```python
from build123d import *

# Parameters (mm, degrees)
F1_DEPTH = 6.35


with BuildPart() as f1:
    # F0 (on Front) → F1 (new body)
    with BuildSketch(Plane.XZ):
        with BuildLine():
            Line((68.58, 18.1031430027), (30.48, 25.4))
            Line((30.48, 25.4), (-30.48, 25.4))
            Line((-30.48, 25.4), (-68.58, 18.1031430027))
            Line((-68.58, 18.1031430027), (-68.58, 17.78))
            ThreePointArc((-68.58, 17.78), (-65.5387583202, 17.5179693185), (-62.5871565312, 16.7396005675))
            Line((-62.5871565312, 16.7396005675), (-61.5696, 17.3270871047))
            Line((-61.5696, 17.3270871047), (-59.9821, 16.4105435523))
            Line((-59.9821, 16.4105435523), (-59.9821, 15.5629211779))
            ThreePointArc((-59.9821, 15.5629211779), (-53.2666224823, 9.0348696172), (-50.8, 0))
            ThreePointArc((-50.8, 0), (-53.2666224823, -9.0348696172), (-59.9821, -15.5629211779))
            Line((-59.9821, -15.5629211779), (-59.9821, -16.4105435523))
            Line((-59.9821, -16.4105435523), (-61.5696, -17.3270871047))
            Line((-61.5696, -17.3270871047), (-62.5871565312, -16.7396005675))
            ThreePointArc((-62.5871565312, -16.7396005675), (-65.5387583202, -17.5179693185), (-68.58, -17.78))
            Line((-68.58, -17.78), (-68.58, -18.1031430027))
            Line((-68.58, -18.1031430027), (-30.48, -25.4))
            Line((-30.48, -25.4), (30.48, -25.4))
            Line((30.48, -25.4), (68.58, -18.1031430027))
            Line((68.58, -18.1031430027), (68.58, -17.78))
            ThreePointArc((68.58, -17.78), (50.8, 0), (68.58, 17.78))
            Line((68.58, 17.78), (68.58, 18.1031430027))
        make_face()
        Polygon((-30.48, -18.4869128953), (-28.8925, -19.4034564477), (-28.8925, -21.2365435523), (-30.48, -22.1530871047), (-32.0675, -21.2365435523), (-32.0675, -19.4034564477), align=None, mode=Mode.SUBTRACT)
        Polygon((-19.05, -15.9469128953), (-17.4625, -16.8634564477), (-17.4625, -18.6965435523), (-19.05, -19.6130871047), (-20.6375, -18.6965435523), (-20.6375, -16.8634564477), align=None, mode=Mode.SUBTRACT)
        Polygon((-48.1514023938, -5.9139128953), (-46.5639023938, -6.8304564477), (-46.5639023938, -8.6635435523), (-48.1514023938, -9.5800871047), (-49.7389023938, -8.6635435523), (-49.7389023938, -6.8304564477), align=None, mode=Mode.SUBTRACT)
        Polygon((0, -18.4869128953), (1.5875, -19.4034564477), (1.5875, -21.2365435523), (0, -22.1530871047), (-1.5875, -21.2365435523), (-1.5875, -19.4034564477), align=None, mode=Mode.SUBTRACT)
        Polygon((30.48, -22.1530871047), (28.8925, -21.2365435523), (28.8925, -19.4034564477), (30.48, -18.4869128953), (32.0675, -19.4034564477), (32.0675, -21.2365435523), align=None, mode=Mode.SUBTRACT)
        Polygon((19.05, -19.6130871047), (17.4625, -18.6965435523), (17.4625, -16.8634564477), (19.05, -15.9469128953), (20.6375, -16.8634564477), (20.6375, -18.6965435523), align=None, mode=Mode.SUBTRACT)
        Polygon((-48.1514023938, 9.5800871047), (-46.5639023938, 8.6635435523), (-46.5639023938, 6.8304564477), (-48.1514023938, 5.9139128953), (-49.7389023938, 6.8304564477), (-49.7389023938, 8.6635435523), align=None, mode=Mode.SUBTRACT)
        Polygon((-19.05, 19.6130871047), (-17.4625, 18.6965435523), (-17.4625, 16.8634564477), (-19.05, 15.9469128953), (-20.6375, 16.8634564477), (-20.6375, 18.6965435523), align=None, mode=Mode.SUBTRACT)
        Polygon((-30.48, 22.1530871047), (-28.8925, 21.2365435523), (-28.8925, 19.4034564477), (-30.48, 18.4869128953), (-32.0675, 19.4034564477), (-32.0675, 21.2365435523), align=None, mode=Mode.SUBTRACT)
        Polygon((19.05, 19.6130871047), (20.6375, 18.6965435523), (20.6375, 16.8634564477), (19.05, 15.9469128953), (17.4625, 16.8634564477), (17.4625, 18.6965435523), align=None, mode=Mode.SUBTRACT)
        Polygon((0, 22.1530871047), (1.5875, 21.2365435523), (1.5875, 19.4034564477), (0, 18.4869128953), (-1.5875, 19.4034564477), (-1.5875, 21.2365435523), align=None, mode=Mode.SUBTRACT)
        Polygon((30.48, 18.4869128953), (28.8925, 19.4034564477), (28.8925, 21.2365435523), (30.48, 22.1530871047), (32.0675, 21.2365435523), (32.0675, 19.4034564477), align=None, mode=Mode.SUBTRACT)
        with BuildLine():
            ThreePointArc((-62.5871565312, 16.7396005675), (-65.5387583202, 17.5179693185), (-68.58, 17.78))
            Line((-68.58, 17.78), (-68.58, 7.3323484187))
            Line((-68.58, 7.3323484187), (-62.23, 3.6661742094))
            Line((-62.23, 3.6661742094), (-62.23, -3.6661742094))
            Line((-62.23, -3.6661742094), (-68.58, -7.3323484187))
            Line((-68.58, -7.3323484187), (-68.58, -17.78))
            ThreePointArc((-68.58, -17.78), (-65.5387583202, -17.5179693185), (-62.5871565312, -16.7396005675))
            Line((-62.5871565312, -16.7396005675), (-63.1571, -16.4105435523))
            Line((-63.1571, -16.4105435523), (-63.1571, -14.5774564477))
            Line((-63.1571, -14.5774564477), (-61.5696, -13.6609128953))
            Line((-61.5696, -13.6609128953), (-59.9821, -14.5774564477))
            Line((-59.9821, -14.5774564477), (-59.9821, -15.5629211779))
            ThreePointArc((-59.9821, -15.5629211779), (-53.2666224823, -9.0348696172), (-50.8, 0))
            ThreePointArc((-50.8, 0), (-53.2666224823, 9.0348696172), (-59.9821, 15.5629211779))
            Line((-59.9821, 15.5629211779), (-59.9821, 14.5774564477))
            Line((-59.9821, 14.5774564477), (-61.5696, 13.6609128953))
            Line((-61.5696, 13.6609128953), (-63.1571, 14.5774564477))
            Line((-63.1571, 14.5774564477), (-63.1571, 16.4105435523))
            Line((-63.1571, 16.4105435523), (-62.5871565312, 16.7396005675))
        make_face()
        with BuildLine():
            Line((-68.58, 7.3323484187), (-68.58, 17.78))
            ThreePointArc((-68.58, 17.78), (-70.259720977, 17.7004784523), (-71.9244167559, 17.4626251338))
            ThreePointArc((-71.9244167559, 17.4626251338), (-86.36, 0), (-71.9244167559, -17.4626251338))
            ThreePointArc((-71.9244167559, -17.4626251338), (-70.259720977, -17.7004784523), (-68.58, -17.78))
            Line((-68.58, -17.78), (-68.58, -7.3323484187))
            Line((-68.58, -7.3323484187), (-74.93, -3.6661742094))
            Line((-74.93, -3.6661742094), (-74.93, 3.6661742094))
            Line((-74.93, 3.6661742094), (-68.58, 7.3323484187))
        make_face()
        Polygon((-74.9877976062, -9.5800871047), (-76.5752976062, -8.6635435523), (-76.5752976062, -6.8304564477), (-74.9877976062, -5.9139128953), (-73.4002976062, -6.8304564477), (-73.4002976062, -8.6635435523), align=None, mode=Mode.SUBTRACT)
        Polygon((-74.9877976062, 9.5800871047), (-73.4002976062, 8.6635435523), (-73.4002976062, 6.8304564477), (-74.9877976062, 5.9139128953), (-76.5752976062, 6.8304564477), (-76.5752976062, 8.6635435523), align=None, mode=Mode.SUBTRACT)
        with BuildLine():
            Line((68.58, -17.78), (68.58, 17.78))
            ThreePointArc((68.58, 17.78), (50.8, 0), (68.58, -17.78))
        make_face()
        Polygon((59.055, -1.8330871047), (57.4675, -0.9165435523), (57.4675, 0.9165435523), (59.055, 1.8330871047), (60.6425, 0.9165435523), (60.6425, -0.9165435523), align=None, mode=Mode.SUBTRACT)
        with BuildLine():
            ThreePointArc((71.9244167559, 17.4626251338), (70.259720977, 17.7004784523), (68.58, 17.78))
            Line((68.58, 17.78), (68.58, -17.78))
            ThreePointArc((68.58, -17.78), (70.259720977, -17.7004784523), (71.9244167559, -17.4626251338))
            ThreePointArc((71.9244167559, -17.4626251338), (82.2838704372, -11.3283862505), (86.36, 0))
            ThreePointArc((86.36, 0), (82.2838704372, 11.3283862505), (71.9244167559, 17.4626251338))
        make_face()
        Polygon((78.105, 1.8330871047), (79.6925, 0.9165435523), (79.6925, -0.9165435523), (78.105, -1.8330871047), (76.5175, -0.9165435523), (76.5175, 0.9165435523), align=None, mode=Mode.SUBTRACT)
        with BuildLine():
            ThreePointArc((-68.58, -17.78), (-70.259720977, -17.7004784523), (-71.9244167559, -17.4626251338))
            Line((-71.9244167559, -17.4626251338), (-68.58, -18.1031430027))
            Line((-68.58, -18.1031430027), (-68.58, -17.78))
        make_face()
        with BuildLine():
            Line((-68.58, 17.78), (-68.58, 18.1031430027))
            Line((-68.58, 18.1031430027), (-71.9244167559, 17.4626251338))
            ThreePointArc((-71.9244167559, 17.4626251338), (-70.259720977, 17.7004784523), (-68.58, 17.78))
        make_face()
        with BuildLine():
            Line((71.9244167559, 17.4626251338), (68.58, 18.1031430027))
            Line((68.58, 18.1031430027), (68.58, 17.78))
            ThreePointArc((68.58, 17.78), (70.259720977, 17.7004784523), (71.9244167559, 17.4626251338))
        make_face()
        with BuildLine():
            ThreePointArc((71.9244167559, -17.4626251338), (70.259720977, -17.7004784523), (68.58, -17.78))
            Line((68.58, -17.78), (68.58, -18.1031430027))
            Line((68.58, -18.1031430027), (71.9244167559, -17.4626251338))
        make_face()
        Polygon((-73.4002976062, 6.8304564477), (-73.4002976062, 8.6635435523), (-74.9877976062, 9.5800871047), (-76.5752976062, 8.6635435523), (-76.5752976062, 6.8304564477), (-74.9877976062, 5.9139128953), align=None)
        Polygon((-76.5752976062, -6.8304564477), (-76.5752976062, -8.6635435523), (-74.9877976062, -9.5800871047), (-73.4002976062, -8.6635435523), (-73.4002976062, -6.8304564477), (-74.9877976062, -5.9139128953), align=None)
        Polygon((-68.58, -7.3323484187), (-68.58, 7.3323484187), (-74.93, 3.6661742094), (-74.93, -3.6661742094), align=None)
        Polygon((-62.23, 3.6661742094), (-68.58, 7.3323484187), (-68.58, -7.3323484187), (-62.23, -3.6661742094), align=None)
        with BuildLine():
            ThreePointArc((-59.9821, 15.5629211779), (-61.260943207, 16.2036973454), (-62.5871565312, 16.7396005675))
            Line((-62.5871565312, 16.7396005675), (-63.1571, 16.4105435523))
            Line((-63.1571, 16.4105435523), (-63.1571, 14.5774564477))
            Line((-63.1571, 14.5774564477), (-61.5696, 13.6609128953))
            Line((-61.5696, 13.6609128953), (-59.9821, 14.5774564477))
            Line((-59.9821, 14.5774564477), (-59.9821, 15.5629211779))
        make_face()
        with BuildLine():
            Line((-61.5696, 17.3270871047), (-62.5871565312, 16.7396005675))
            ThreePointArc((-62.5871565312, 16.7396005675), (-61.260943207, 16.2036973454), (-59.9821, 15.5629211779))
            Line((-59.9821, 15.5629211779), (-59.9821, 16.4105435523))
            Line((-59.9821, 16.4105435523), (-61.5696, 17.3270871047))
        make_face()
        Polygon((-46.5639023938, 6.8304564477), (-46.5639023938, 8.6635435523), (-48.1514023938, 9.5800871047), (-49.7389023938, 8.6635435523), (-49.7389023938, 6.8304564477), (-48.1514023938, 5.9139128953), align=None)
        Polygon((-46.5639023938, -8.6635435523), (-46.5639023938, -6.8304564477), (-48.1514023938, -5.9139128953), (-49.7389023938, -6.8304564477), (-49.7389023938, -8.6635435523), (-48.1514023938, -9.5800871047), align=None)
        with BuildLine():
            Line((-63.1571, -16.4105435523), (-62.5871565312, -16.7396005675))
            ThreePointArc((-62.5871565312, -16.7396005675), (-61.260943207, -16.2036973454), (-59.9821, -15.5629211779))
            Line((-59.9821, -15.5629211779), (-59.9821, -14.5774564477))
            Line((-59.9821, -14.5774564477), (-61.5696, -13.6609128953))
            Line((-61.5696, -13.6609128953), (-63.1571, -14.5774564477))
            Line((-63.1571, -14.5774564477), (-63.1571, -16.4105435523))
        make_face()
        with BuildLine():
            ThreePointArc((-59.9821, -15.5629211779), (-61.260943207, -16.2036973454), (-62.5871565312, -16.7396005675))
            Line((-62.5871565312, -16.7396005675), (-61.5696, -17.3270871047))
            Line((-61.5696, -17.3270871047), (-59.9821, -16.4105435523))
            Line((-59.9821, -16.4105435523), (-59.9821, -15.5629211779))
        make_face()
        Polygon((-17.4625, 16.8634564477), (-17.4625, 18.6965435523), (-19.05, 19.6130871047), (-20.6375, 18.6965435523), (-20.6375, 16.8634564477), (-19.05, 15.9469128953), align=None)
        Polygon((-17.4625, -18.6965435523), (-17.4625, -16.8634564477), (-19.05, -15.9469128953), (-20.6375, -16.8634564477), (-20.6375, -18.6965435523), (-19.05, -19.6130871047), align=None)
        Polygon((17.4625, -16.8634564477), (17.4625, -18.6965435523), (19.05, -19.6130871047), (20.6375, -18.6965435523), (20.6375, -16.8634564477), (19.05, -15.9469128953), align=None)
        Polygon((20.6375, 16.8634564477), (20.6375, 18.6965435523), (19.05, 19.6130871047), (17.4625, 18.6965435523), (17.4625, 16.8634564477), (19.05, 15.9469128953), align=None)
    extrude(amount=F1_DEPTH)


solid = f1.part
```
Here's how the part is built. I have some questions about the finished solid (model axes, mm). Give positions to 0.01 mm unless a question says otherwise; leave off trailing zeros. Loops run counter-clockwise (first coordinate to the right, second up) from the corner with the lowest first, then second, coordinate; pieces in that order, holes last. Notation, with made-up numbers: M -39,-34.75 L -35,-34.75 A14 cw -35,-17.75 Z; hole C 19.25,51.5 d4. An arc over 180 degrees is marked long. Return JSON: item names as keys, results as strings.
Item 1: Imagine slicing it at A-A on y = -3. State how many separate pieces and enclosed holes the cut face has, then the cut area to 3 significant figures.
A:
{"separate pieces": "1", "enclosed holes": "8", "area": "7,340 mm^2"}
Item 2: Thinking about a two-plate mould opening in Z: for faces 1 (the flat face through (0, -3, -25.4)), 2 (the flat face through (0, -3, 25.4)), 3 (the flat face through (-1, -6.35, 0)), which applies, released by +Z, released by -Z, zero draft, split by the parting line, or undercut?
A:
{"face 1": "released by -Z", "face 2": "released by +Z", "face 3": "zero draft"}
Item 3: Imagine slicing it at C-C on z = -11. List the corners of the cut face in (x, y) for me, then the cut area to 3 significant figures.
A:
{"outline": "M -82.55,-6.35 L 82.55,-6.35 L 82.55,0 L -82.55,0 Z", "area": "1,050 mm^2"}
Item 4: Imagine slicing it at B-B on x = 38.5. List the corners of the cut face in (y, z) for me, then the cut area to 3 significant figures.
A:
{"outline": "M -6.35,-23.86 L 0,-23.86 L 0,23.86 L -6.35,23.86 Z", "area": "303 mm^2"}
Item 5: Please list where these lines run through material, in increasing order: line 1 (X direction, y = -0.5, z = 1); line 2 (Z direction, x = 77.5, y = -5.5); line 3 (Z direction, x = 59, y = -3.75).
A:
{"line 1": "x = -86.33 to 57.61, 60.5 to 76.66, 79.55 to 86.33", "line 2": "z = -15.38 to -1.48, 1.48 to 15.38", "line 3": "z = -19.94 to -1.8, 1.8 to 19.94"}
